Geometry check sheet. Reference: the model listing, model coordinates, mm. A direction names the side the tool comes from. Give positions to 0.01 mm unless a question says otherwise; leave off trailing zeros. Write each loop counter-clockwise with the first axis right and the second up, starting at its lowest first coordinate (ties: lowest second). Pieces come first, ordered by that corner, then holes.
(1) Mould release check, pull along Z, two halves, no side actions. Record for faces 1 (the flat face through (0, 24, 0)), 2 (the flat face through (0, 24, -28)), 3 (the flat face through (0, 35, 3)): +Z half, -Z half, draft (parallel to the pull), parting line (faces both ways), or undercut.
(2) Cross-section at D-D (y = 34). Record the boundary of the cut face in (x, z) (3 decimals), and give its area (3 significant figures).
(3) Cross-section at B-B (y = 7). Record the boundary of the cut face in (x, z), and give its area (3 significant figures).
(4) Tool access check on faces 4 (the flat face through (-18, 20, -25)), 5 (the flat face through (-16, 12, 0)), 6 (the cylindrical face through (-19, 24, -39)), 7 (the flat face through (0, 40, -22)), 8 (the flat face through (-19, 28, -31)). Record the directions out of +Z, -Z, +X, -X, +Y, -Y that give a thin tool (end or side, any length) a straight path to the whole face; none if there is none.
(5) Cross-section at A-A (z = 0.5). Record the boundary of the cut face in (x, y).
(6) Thickness scan on line 1 along X through (y, z) = (22, 24) (3 decimals); line 2 along X through (y, z) = (10, -8.5); line 3 along Y through (x, z) = (19.05, -35). Record the ranges inside material, lowest first.
(7) Cross-section at C-C (x = -6). Record the boundary of the cut face in (y, z), and give its area (3 significant figures).
(8) Depth check by flat-ended pin: P1, Ø0.8, axis at x = 19, z = -28.5, coming from the -Y side; P2, Ø1, axis at x = 7.5, z = 8.5, coming from the -Y side; P3, Ø6, axis at x = -11.5, y = 35.5, coming from the -Z side. Enter the tip coordinate at first touch or a pass-through.
Autodesk Fusion 360 part; units mm, degrees
sketch "Sketch1" plane through (0, 0, 0) normal (0, 1, 0) x (1, 0, 0)
  line L0 (-16, 24) -> (16, 24)
  line L1 (16, 24) -> (16, -24)
  line L2 (16, -24) -> (-16, -24)
  line L3 (-16, -24) -> (-16, 24)
  line L4 (-16, 24) -> (16, -24) construction
  line L5 (16, 24) -> (-16, -24) construction
  circle A0 centre (-16, 24) radius 2.5
  circle A1 centre (16, 24) radius 2.5
  circle A2 centre (-16, -24) radius 2.5
  circle A3 centre (16, -24) radius 2.5
  circle A4 centre (-16, -24) radius 4
  circle A5 centre (16, -24) radius 4
  circle A6 centre (16, 24) radius 4
  circle A7 centre (-16, 24) radius 4
  line L6 (-16, 24) -> (-16, 28)
  line L7 (-16, 28) -> (16, 28)
  line L8 (-16, 24) -> (-20, 24)
  line L9 (-16, -24) -> (-20, -24)
  line L10 (-20, 24) -> (-20, -24)
  line L11 (-16, -24) -> (-16, -28)
  line L12 (-16, -28) -> (16, -28)
  line L13 (16, -24) -> (20, -24)
  line L14 (20, -24) -> (20, 24)
  dimension "d1" = 32
  dimension "d2" = 48
  dimension "d3" = 5
  dimension "d4" = 5
  dimension "d5" = 5
  dimension "d6" = 5
  dimension "d7" = 8
  dimension "d8" = 8
  dimension "d9" = 8
  dimension "d10" = 8
extrude "Extrude1" add sketch "Sketch1" along normal blind 8 contours L0 A0 A7 L6 | L0 L3 A0 A7 | L3 A0 A7 L8 | A0 A7 L6 L8 | L0 A6 A7 L7 | L0 L1 L2 L3 A4 A5 A6 A7 | L3 A4 A7 L10 | L0 L1 A1 A6 | L0 L1 A1 A6 | L2 L3 A2 A4 | L3 A2 A4 L9 | A2 A4 L9 L11 | L1 A5 A6 L14 | L2 A2 A4 L11 | L2 A4 A5 L12 | L1 A3 A5 L13 | L1 L2 A3 A5 | L2 A3 A5 L13
sketch "Sketch2" plane through (0, 0, 0) normal (0, -1, 0) x (1, 0, 0)
  circle A0 centre (16, 24) radius 2.5
  circle A1 centre (-16, 24) radius 2.5
  circle A2 centre (-16, -24) radius 2.5
  circle A3 centre (16, -24) radius 2.5
  arc A4 (-20, -24) -> (-16, -28) centre (-16, -24) ccw
  line L0 (-16, -28) -> (16, -28)
  arc A5 (16, -28) -> (20, -24) centre (16, -24) ccw
  line L1 (20, -24) -> (20, 24)
  arc A6 (20, 24) -> (16, 28) centre (16, 24) ccw
  line L2 (16, 28) -> (-16, 28)
  arc A7 (-16, 28) -> (-20, 24) centre (-16, 24) ccw
  line L3 (-20, 24) -> (-20, -24)
  circle A8 centre (-16, -24) radius 3.2
  circle A9 centre (16, -24) radius 3.2
  circle A10 centre (-16, 24) radius 3.2
  circle A11 centre (16, 24) radius 3.2
  dimension "d13" = 6.4
  dimension "d14" = 6.4
  dimension "d15" = 6.4
  dimension "d16" = 6.4
extrude "Extrude2" cut sketch "Sketch2" against normal blind 2.5 contours A8 | A9 | A10 | A11
sketch "Sketch3" plane through (0, 8, 0) normal (0, 1, 0) x (-1, 0, 0)
  circle A0 centre (-16, 24) radius 2.5
  circle A1 centre (16, 24) radius 2.5
  circle A2 centre (16, -24) radius 2.5
  circle A3 centre (-16, -24) radius 2.5
  arc A4 (16, -28) -> (20, -24) centre (16, -24) ccw
  line L0 (20, -24) -> (20, 24)
  arc A5 (20, 24) -> (16, 28) centre (16, 24) ccw
  line L1 (16, 28) -> (-16, 28)
  arc A6 (-16, 28) -> (-20, 24) centre (-16, 24) ccw
  line L2 (-20, 24) -> (-20, -24)
  arc A7 (-20, -24) -> (-16, -28) centre (-16, -24) ccw
  line L3 (-16, -28) -> (16, -28)
  circle A8 centre (16, -24) radius 3.125
  circle A9 centre (-16, -24) radius 3.125
  circle A10 centre (16, 24) radius 3.125
  dimension "d19" = 6.25
  dimension "d20" = 6.25
  dimension "d21" = 6.25
extrude "Extrude3" add sketch "Sketch3" along normal blind 35 contours A4 L0 A5 L1 A6 L2 A7 L3
extrude "Extrude4" add 1 faces at (5.0453, 43, 7.366) along direction (0, 1, 0) blind 5
sketch "Sketch4" plane through (0, 0, 28) normal (0, 0, 1) x (1, 0, 0)
  line L0 (-16, 0) -> (16, 0)
  line L1 (16, 0) -> (16, 48)
  line L2 (16, 48) -> (-16, 48)
  line L3 (-16, 48) -> (-16, 0)
  line L4 (-18, 45) -> (18, 45)
  line L5 (18, 45) -> (18, 35)
  line L6 (18, 35) -> (-18, 35)
  line L7 (-18, 35) -> (-18, 45)
  line L8 (-18, 45) -> (18, 35) construction
  line L9 (18, 45) -> (-18, 35) construction
  point P0 (0, 40)
extrude "Extrude5" cut sketch "Sketch4" against normal blind 50 contours L3 L4 L6 L7 | L1 L3 L4 L6 | L1 L4 L5 L6
sketch "Sketch5" plane through (-20, 0, 0) normal (-1, 0, 0) x (0, 0, 1)
  line L0 (-24, 0) -> (24, 0)
  line L1 (24, 0) -> (24, 48)
  line L2 (24, 48) -> (-24, 48)
  line L3 (-24, 48) -> (-24, 0)
  line L4 (-24, 0) -> (-24, 24)
  line L5 (-24, 24) -> (-35, 24)
  circle A0 centre (-35, 24) radius 1.75
  circle A1 centre (-35, 24) radius 4
  line L6 (-35, 24) -> (-35, 28)
  line L7 (-35, 24) -> (-35, 20)
  line L8 (-35, 20) -> (-24, 20)
  line L9 (-35, 28) -> (-24, 28)
  dimension "d28" = 3.5
  dimension "d29" = 8
extrude "Extrude6" add sketch "Sketch5" against normal blind 2.5 contours L3 L4 L5 A1 L8 | L3 L5 A1 L9 | L5 A0 A1 L7 | A0 A1 L6 L7 | L5 A0 A1 L6
sketch "Sketch6" plane through (20, 0, 0) normal (1, 0, 0) x (0, 0, -1)
  line L0 (-24, 0) -> (24, 0)
  line L1 (24, 0) -> (24, 48)
  line L2 (24, 48) -> (-24, 48)
  line L3 (-24, 48) -> (-24, 0)
  line L4 (24, 24) -> (35, 24)
  circle A0 centre (35, 24) radius 1.75
  circle A1 centre (35, 24) radius 4
  line L5 (35, 24) -> (35, 28)
  line L6 (35, 24) -> (35, 20)
  line L7 (35, 20) -> (24, 20)
  line L8 (35, 28) -> (24, 28)
  dimension "d32" = 3.5
extrude "Extrude7" add sketch "Sketch6" against normal blind 2.5 contours L1 L4 A1 L7 | L1 L4 A1 L8 | A0 A1 L5 L6 | L4 A0 A1 L6 | L4 A0 A1 L5
sketch "Sketch7" plane through (0, 0, 0) normal (0, -1, 0) x (1, 0, 0)
  circle A0 centre (16, 24) radius 3.2
  circle A1 centre (-16, -24) radius 3.2
  circle A2 centre (-16, 24) radius 3.2
  circle A3 centre (16, -24) radius 3.2
  arc A4 (-20, -24) -> (-16, -28) centre (-16, -24) ccw
  line L0 (-16, -28) -> (16, -28)
  arc A5 (16, -28) -> (20, -24) centre (16, -24) ccw
  line L1 (20, -24) -> (20, 24)
  arc A6 (20, 24) -> (16, 28) centre (16, 24) ccw
  line L2 (16, 28) -> (-16, 28)
  arc A7 (-16, 28) -> (-20, 24) centre (-16, 24) ccw
  line L3 (-20, 24) -> (-20, -24)
  line L4 (16, -18) -> (-16, -18)
  line L5 (-16, -18) -> (-16, 18)
  line L6 (-16, 18) -> (16, 18)
  line L7 (16, 18) -> (16, -18)
  line L8 (16, -18) -> (-16, 18) construction
  line L9 (-16, -18) -> (16, 18) construction
extrude "Extrude8" cut sketch "Sketch7" against normal blind 24 contours L4 L5 L6 L7
Reply:
1. face 1: undercut
1. face 2: -Z half
1. face 3: draft
2. outline: (-20, -24) arc R4 ccw to (-16, -28) - (16, -28) arc R4 ccw to (20, -24) - (20, 24) arc R4 ccw to (16, 28) - (-16, 28) arc R4 ccw to (-20, 24) - close; hole circle Ø6.25 at (-16, -24); hole circle Ø6.25 at (-16, 24); hole circle Ø6.25 at (16, -24); hole circle Ø5 at (16, 24)
2. area: 2,110 mm2
3. outline: (-20, -24) arc R4 ccw to (-16, -28) - (16, -28) arc R4 ccw to (20, -24) - (20, 24) arc R4 ccw to (16, 28) - (-16, 28) arc R4 ccw to (-20, 24) - close; hole circle Ø5 at (-16, -24); hole circle Ø5 at (-16, 24); hole (-16, -18) - (16, -18) - (16, 18) - (-16, 18) - close; hole circle Ø5 at (16, -24); hole circle Ø5 at (16, 24)
3. area: 996 mm2
4. face 4: none
4. face 5: -Y
4. face 6: -Z, +X, -X
4. face 7: +Z
4. face 8: -Z, -X, +Y
5. outline: (-20, 0) - (-16, 0) - (-16, 24) - (16, 24) - (16, 0) - (20, 0) - (20, 48) - (-20, 48) - close; hole (-18, 35) - (18, 35) - (18, 45) - (-18, 45) - close
6. line 1: x = -20 to -19.125, -12.875 to 13.5, 18.5 to 20
6. line 2: x = -20 to -16, 16 to 20
6. line 3: y = 20 to 22.25, 25.75 to 28
7. outline: (0, -28) - (48, -28) - (48, 28) - (45, 28) - (45, -22) - (35, -22) - (35, 28) - (0, 28) - (0, 18) - (24, 18) - (24, -18) - (0, -18) - close
7. area: 1,320 mm2
8. P1: stops at y = 20
8. P2: stops at y = 24
8. P3: stops at z = -28
